Autodesk Inventor part; units mm, degrees
ref_plane "YZ Plane" through (0, 0, 0) normal (1, 0, 0) x (0, 1, 0)
ref_plane "XZ Plane" through (0, 0, 0) normal (0, 1, 0) x (-1, 0, 0)
ref_plane "XY Plane" through (0, 0, 0) normal (0, 0, 1) x (1, 0, 0)
sketch "Sketch1" plane through (0, 0, 0) normal (0, 0, 1) x (1, 0, 0)
  line L0 (0, 0) -> (44, 0)
  line L1 (44, 0) -> (44, 9)
  line L2 (32, 12) -> (12, 12)
  line L3 (0, 9) -> (0, 0)
  line L4 (12, 12) -> (12, 9)
  line L5 (12, 9) -> (0, 9)
  line L6 (32, 12) -> (32, 9)
  line L7 (32, 9) -> (44, 9)
  dimension "d6" = 44
  dimension "d7" = 3
  dimension "d8" = 3
  dimension "d9" = 12
  dimension "d10" = 12
  dimension "d11" = 9
  dimension "d12" = 9
  dimension "d13" = 12
extrude "Extrusion1" add sketch "Sketch1" along normal blind 6
sketch "Sketch2" plane through (0, 0, 0) normal (0, 0, -1) x (-1, 0, 0)
  line L0 (-32, 12) -> (-12, 12)
  line L1 (0, 0) -> (-44, 0)
  line L2 (-32, 12) -> (-12, 12)
  line L3 (-12, 12) -> (-12, 0)
  line L4 (-12, 0) -> (-32, 0)
  line L5 (-32, 0) -> (-32, 12)
extrude "Extrusion2" add sketch "Sketch2" along normal blind 6
sketch "Sketch3" plane through (0, 0, 0) normal (0, 0, -1) x (-1, 0, 0)
  circle A0 centre (-6, 4.5) radius 1.725
  line L0 (-12, 9) -> (0, 9)
  line L1 (0, 9) -> (0, 0)
  circle A1 centre (-38, 4.5) radius 1.725
  line L2 (-32, 0) -> (-44, 0)
  line L3 (-44, 0) -> (-44, 9)
  dimension "d18" = 3.45
  dimension "d19" = 4.5
  dimension "d20" = 6
  dimension "d21" = 3.45
  dimension "d22" = 4.5
  dimension "d23" = 6
extrude "Extrusion3" cut sketch "Sketch3" against normal blind 3
sketch "Sketch4" plane through (0, 0, 6) normal (0, 0, 1) x (1, 0, 0)
  circle A0 centre (6, 4.5) radius 3
  line L0 (12, 9) -> (0, 9)
  line L1 (0, 9) -> (0, 0)
  circle A1 centre (38, 4.5) radius 1.725
  circle A2 centre (38, 4.5) radius 3
  dimension "d26" = 6
  dimension "d27" = 4.5
  dimension "d28" = 6
  dimension "d29" = 6
extrude "Extrusion4" cut sketch "Sketch4" against normal blind 3 contours A0 | A1 | A2
fillet "Fillet1" radius 1.5 2 edges at (22, 12, 6) (22, 12, -6)
equation "\"d8\" = d7"
equation "\"d10\" = d9"
equation "\"d12\" = d11"
properties part number "beam44mm"
Check sheet for the modelled part. Datum: model origin and axes. Units: mm. A direction names the side the tool comes from. Coordinates: 2 decimals unless noted, no trailing zeros. Loops run counter-clockwise (first coordinate to the right, second up) from the corner with the lowest first, then second, coordinate; pieces in that order, holes last. Notation, with made-up numbers: (6.5, -9) -> (58.5, -9) arc R35 cw to (58.5, 28) -> close; hole circle Ø7 at (24, 18.5). An arc over 180 degrees is marked (long way). Write item = value, one per line. Start each with the question number.
1. Tool access check on faces 1 (the cylindrical face through (35, 4.6, 4.5)), 2 (the flat face through (6, 9, 3)), 3 (the flat face through (6, 7, 0)). Record the directions out of +Z, -Z, +X, -X, +Y, -Y that give a thin tool (end or side, any length) a straight path to the whole face; none if there is none.
2. Section check C-C on z = 0.75. Record the cut outline in (x, y) (3 decimals), then the cut area to 3 significant figures.
3. Material ranges on line 1 (Y direction, x = 6, z = 2.25) (3 decimals); line 2 (Y direction, x = 38, z = 5.05); line 3 (X direction, y = 5.5, z = 1.5), recorded low to high.
4. Draft check along X on faces 4 (the flat face through (44, 4, 3)), 5 (the flat face through (38, 7, 0)), 6 (the cylindrical face through (39.723, 4.576, 1.479)). Enter one of: released by +X, released by -X, zero draft, split by the parting line, or undercut.
5. Depth check by flat-ended pin: P1, Ø3, axis at y = 9, z = -3.5, coming from the -X side; P2, Ø2.5, axis at x = 39.5, y = 5.5, coming from the -Z side; P3, Ø6.5, axis at x = 4.5, z = 3.5, coming from the +Y side. Enter the tip coordinate at first touch or a pass-through.
6. Section check B-B on x = 38. Record the cut outline in (y, z) (3 decimals).
7. Section check A-A on y = 4.5. Record the cut outline in (x, z) (3 decimals).
8. Section check D-D on y = 8. Record the cut outline in (x, z).
Responses:
q1.face_1 = +Z
q1.face_2 = +Z, -Z, -X, +Y
q1.face_3 = -Z, -X, +Y, -Y
q2.outline = (0, 0) -> (44, 0) -> (44, 9) -> (32, 9) -> (32, 12) -> (12, 12) -> (12, 9) -> (0, 9) -> close; hole circle Ø3.45 at (6, 4.5); hole circle Ø3.45 at (38, 4.5)
q2.area = 437 mm2
q3.line_1 = 0 to 2.775, 6.225 to 9
q3.line_2 = 0 to 1.5, 7.5 to 9
q3.line_3 = 0 to 4.59, 7.41 to 36.59, 39.41 to 44
q4.face_4 = released by +X
q4.face_5 = zero draft
q4.face_6 = undercut
q5.P1 = 12
q5.P2 = 0
q5.P3 = 9
q6.outline = (0, 0) -> (2.775, 0) -> (2.775, 3) -> (1.5, 3) -> (1.5, 6) -> (0, 6) -> close; (6.225, 0) -> (9, 0) -> (9, 6) -> (7.5, 6) -> (7.5, 3) -> (6.225, 3) -> close
q7.outline = (0, 0) -> (4.275, 0) -> (4.275, 3) -> (3, 3) -> (3, 6) -> (0, 6) -> close; (7.725, 0) -> (12, 0) -> (12, -6) -> (32, -6) -> (32, 0) -> (36.275, 0) -> (36.275, 3) -> (35, 3) -> (35, 6) -> (9, 6) -> (9, 3) -> (7.725, 3) -> close; (39.725, 0) -> (44, 0) -> (44, 6) -> (41, 6) -> (41, 3) -> (39.725, 3) -> close
q8.outline = (0, 0) -> (12, 0) -> (12, -6) -> (32, -6) -> (32, 0) -> (44, 0) -> (44, 6) -> (0, 6) -> close
